Can you work these out from the model? Positions are in its coordinate system, mm. A direction names the side the tool comes from. Give positions to 0.01 mm unless a question says otherwise; leave off trailing zeros. Loops run counter-clockwise (first coordinate to the right, second up) from the corner with the lowest first, then second, coordinate; pieces in that order, holes last. Notation, with made-up numbers: (6, 81) -> (54, 81) arc R26 cw to (54, 104) -> close; hole circle Ø1 at (-38.75, 33). An arc over 180 degrees is marked (long way). Use CSV: the item, a comma, the result in double quotes.
from build123d import *

# Parameters (mm, degrees)
SKETCH2_W           = 88.9
SKETCH2_H           = 25.4
SKETCH2_R           = 3.175
SKETCH2_R_2         = 6.35
BOSS_EXTRUDE1_DEPTH = 6.35
SKETCH3_R           = 5.08
CUT_EXTRUDE1_DEPTH  = 93.675198948
SKETCH4_R           = 5.08
SKETCH4_R_2         = 3.175
BOSS_EXTRUDE2_DEPTH = 12.7
SKETCH5_R           = 5.08
SKETCH5_R_2         = 3.175
BOSS_EXTRUDE3_DEPTH = 9.525


with BuildPart() as part:
    # Sketch2 → Boss-Extrude1 (new body)
    with BuildSketch(Plane(origin=(0, 0, 0), x_dir=(1, 0, 0), z_dir=(0, 1, 0))):
        with Locations((0, 12.7)):
            Rectangle(SKETCH2_W, SKETCH2_H)
        with Locations(Location((-31.75, 12.7, 0), (0, 0, 270))):
            Circle(SKETCH2_R, mode=Mode.SUBTRACT)
        with Locations(Location((0, 12.7, 0), (0, 0, 270))):
            Circle(SKETCH2_R_2, mode=Mode.SUBTRACT)
        with Locations(Location((31.75, 12.7, 0), (0, 0, 270))):
            Circle(SKETCH2_R, mode=Mode.SUBTRACT)
    extrude(amount=BOSS_EXTRUDE1_DEPTH)

    # Sketch3 → Cut-Extrude1 (cut, through all)
    with BuildSketch(Plane.ZY.offset(44.45)):
        with Locations((0, 6.35)):
            Circle(SKETCH3_R)
    extrude(amount=-CUT_EXTRUDE1_DEPTH, mode=Mode.SUBTRACT)

    # Sketch4 → Boss-Extrude2 (add)
    with BuildSketch(Plane.ZY.offset(44.45)):
        with Locations((0, 6.35)):
            Circle(SKETCH4_R)
        with Locations((0, 6.35)):
            Circle(SKETCH4_R_2, mode=Mode.SUBTRACT)
    boss_extrude2 = extrude(amount=-BOSS_EXTRUDE2_DEPTH)

    # Mirror1: Boss-Extrude2 across plane
    add(boss_extrude2.mirror(Plane(origin=(0, 0, 0), x_dir=(0, 0, 1), z_dir=(1, 0, 0))))

    # Sketch5 → Boss-Extrude3 (add, symmetric)
    with BuildSketch(Plane(origin=(0, 0, 0), x_dir=(0, 0, -1), z_dir=(1, 0, 0))):
        with Locations((0, 6.35)):
            Circle(SKETCH5_R)
        with Locations(Location((0, 6.35, 0), (0, 0, 180))):
            Circle(SKETCH5_R_2, mode=Mode.SUBTRACT)
    extrude(amount=BOSS_EXTRUDE3_DEPTH, both=True)


solid = part.part
(1) If we section it at A-A, the plane x = 0: Write out the boundary of the cut face in (y, z) (3 decimals).
Answer sheet:
outline,"(0, -25.4) -> (6.35, -25.4) -> (6.35, -19.05) -> (0, -19.05) -> close; (0, -6.35) -> (6.35, -6.35) -> (6.35, -5.08) arc R5.08 ccw (long way) to (1.27, 0) -> (0, 0) -> close; hole circle Ø6.35 at (6.35, 0)"
(2) If we section it at C-C, the plane y = 8.75: Write out the boundary of the cut face in (x, z) (3 decimals), then the cut area to 3 significant figures.
Answer sheet:
outline,"(-44.45, -4.477) -> (-31.75, -4.477) -> (-31.75, -2.079) -> (-44.45, -2.079) -> close; (-44.45, 2.079) -> (-31.75, 2.079) -> (-31.75, 4.477) -> (-44.45, 4.477) -> close; (-9.525, -4.477) -> (9.525, -4.477) -> (9.525, -2.079) -> (-9.525, -2.079) -> close; (-9.525, 2.079) -> (9.525, 2.079) -> (9.525, 4.477) -> (-9.525, 4.477) -> close; (31.75, -4.477) -> (44.45, -4.477) -> (44.45, -2.079) -> (31.75, -2.079) -> close; (31.75, 2.079) -> (44.45, 2.079) -> (44.45, 4.477) -> (31.75, 4.477) -> close"
area,"213 mm2"
(3) Will these pins go through, and if not, where does the flat tip stop? pin 1 Ø5 at (x, y) = (-1.5, 3) entering from +Z; pin 2 Ø1.5 at (x, z) = (-4, -4) entering from -Y; pin 3 Ø8 at (x, z) = (25, -8.5) entering from +Y; pin 4 Ø10 at (x, z) = (3, -15) entering from +Y.
Answer sheet:
pin 1,"stops at z = 5.01"
pin 2,"stops at y = 0"
pin 3,"stops at y = 6.35"
pin 4,"stops at y = 6.35"
(4) Which directions (+Z, -Z, +X, -X, +Y, -Y) give clear straight access to the entire face, cutting with the end or side of a thin tool? Please do faces 1 (the face through (-31.75, 3, 0)), 2 (the face through (1.907, 3.131, -6.643)), 3 (the face through (-1, 6.35, -20)).
Answer sheet:
face 1,"+Z, +Y"
face 2,"+Y, -Y"
face 3,"-Z, +X, -X, +Y"
(5) If we section it at B-B, the plane z = -12.7: Write out the boundary of the cut face in (x, y) (3 decimals).
Answer sheet:
outline,"(-44.45, 0) -> (-34.925, 0) -> (-34.925, 6.35) -> (-44.45, 6.35) -> close; (-28.575, 0) -> (-6.35, 0) -> (-6.35, 6.35) -> (-28.575, 6.35) -> close; (6.35, 0) -> (28.575, 0) -> (28.575, 6.35) -> (6.35, 6.35) -> close; (34.925, 0) -> (44.45, 0) -> (44.45, 6.35) -> (34.925, 6.35) -> close"
(6) We'd pull the mould along Z, two halves only. Please class faces 4 (the face through (-1, 0, -21)), 5 (the face through (-38.19, 9.82, 3.71)), 6 (the face through (20.482, 2.798, -3.631)), 7 (the face through (28.65, 3.13, -13.39)): released by +Z, released by -Z, zero draft, split by the parting line, or undercut.
Answer sheet:
face 4,"zero draft"
face 5,"split by the parting line"
face 6,"released by +Z"
face 7,"undercut"
(7) If I drill on L1, parallel to X at y = 3.5, z = -12.7 (3 decimals); L2, parallel to X at y = 2.25, z = 2 (3 decimals); L3, parallel to X at y = 2.75, z = -13.5, over which ranges is the centre line in solid material (lowest first)? Write a range as from..to.
Answer sheet:
L1,"x = -44.45..-34.925, -28.575..-6.35, 6.35..28.575, 34.925..44.45"
L2,"x = -44.45..-31.75, -9.525..9.525, 31.75..44.45"
L3,"x = -44.45..-34.82, -28.68..-6.3, 6.3..28.68, 34.82..44.45"
(8) If we section it at D-D, the plane z = 1.5: Give the number of separate pieces and of enclosed holes in the cut face, then the cut area to 3 significant figures.
Answer sheet:
separate pieces,"6"
enclosed holes,"0"
area,"183 mm2"
